```python
from build123d import *

# Parameters (mm, degrees)
SKETCH1_W           = 596.9
SKETCH1_H           = 12.7
BOSS_EXTRUDE1_DEPTH = 6.35
SKETCH3_W           = 37.846
SKETCH3_H           = 6.35
BOSS_EXTRUDE2_DEPTH = 3.175
SKETCH4_R           = 3.429
SKETCH4_R_2         = 4.8895
CUT_EXTRUDE1_DEPTH  = 299.669467179
SKETCH5_R           = 4.9784
CUT_EXTRUDE2_DEPTH  = 299.669467179
CUT_EXTRUDE3_DEPTH  = 299.669467179


with BuildPart() as part:
    # Sketch1 → Boss-Extrude1 (new body)
    with BuildSketch(Plane.XY):
        Rectangle(SKETCH1_W, SKETCH1_H)
    extrude(amount=BOSS_EXTRUDE1_DEPTH)

    # Sketch3 → Boss-Extrude2 (add)
    with BuildSketch(Plane(origin=(0, 6.35, 0), x_dir=(1, 0, 0), z_dir=(0, 1, 0))):
        with Locations((-199.093666667, -3.175)):
            Rectangle(SKETCH3_W, SKETCH3_H)
        with Locations((-99.610333333, -3.175)):
            Rectangle(SKETCH3_W, SKETCH3_H)
        with Locations((-0.127, -3.175)):
            Rectangle(SKETCH3_W, SKETCH3_H)
        with Locations((99.483333333, -3.175)):
            Rectangle(SKETCH3_W, SKETCH3_H)
        with Locations((198.966666751, -3.175)):
            Rectangle(SKETCH3_W, SKETCH3_H)
    boss_extrude2 = extrude(amount=BOSS_EXTRUDE2_DEPTH)

    # Mirror1: Boss-Extrude2 across plane
    add(boss_extrude2.mirror(Plane.ZX))

    # Sketch4 → Cut-Extrude1 (cut, through all)
    with BuildSketch(Plane(origin=(0, 0, 0), x_dir=(-1, 0, 0), z_dir=(0, 0, -1))):
        with Locations((-288.925, 0)):
            Circle(SKETCH4_R)
        with Locations((-244.475, 0)):
            Circle(SKETCH4_R)
        with Locations((-266.7, 0)):
            Circle(SKETCH4_R_2)
    cut_extrude1 = extrude(amount=-CUT_EXTRUDE1_DEPTH, mode=Mode.SUBTRACT)

    # Mirror2: Cut-Extrude1 across plane
    add(cut_extrude1.mirror(Plane(origin=(0, 0, 0), x_dir=(0, 0, 1), z_dir=(1, 0, 0))), mode=Mode.SUBTRACT)

    # Sketch5 → Cut-Extrude2 (cut, through all)
    with BuildSketch(Plane(origin=(0, 0, 0), x_dir=(-1, 0, 0), z_dir=(0, 0, -1))):
        with Locations((-266.7, 0)):
            Circle(SKETCH5_R)
    extrude(amount=-CUT_EXTRUDE2_DEPTH, mode=Mode.SUBTRACT)

    # Sketch6 → Cut-Extrude3 (cut, through all)
    with BuildSketch(Plane.XY.offset(6.35)):
        with BuildLine():
            Line((-208.618666667, 3.81), (-189.568666667, 3.81))
            ThreePointArc((-189.568666667, 3.81), (-185.758666667, 0), (-189.568666667, -3.81))
            Line((-189.568666667, -3.81), (-208.618666667, -3.81))
            ThreePointArc((-208.618666667, -3.81), (-212.428666667, 0), (-208.618666667, 3.81))
        make_face()
        with BuildLine():
            Line((-109.135333333, 3.81), (-90.085333333, 3.81))
            ThreePointArc((-90.085333333, 3.81), (-86.275333333, 0), (-90.085333333, -3.81))
            Line((-90.085333333, -3.81), (-109.135333333, -3.81))
            ThreePointArc((-109.135333333, -3.81), (-112.945333333, 0), (-109.135333333, 3.81))
        make_face()
        with BuildLine():
            Line((-9.652, 3.81), (9.398, 3.81))
            ThreePointArc((9.398, 3.81), (13.208, 0), (9.398, -3.81))
            Line((9.398, -3.81), (-9.652, -3.81))
            ThreePointArc((-9.652, -3.81), (-13.462, 0), (-9.652, 3.81))
        make_face()
        with BuildLine():
            Line((89.831333333, 3.81), (108.881333333, 3.81))
            ThreePointArc((108.881333333, 3.81), (112.691333333, 0), (108.881333333, -3.81))
            Line((108.881333333, -3.81), (89.831333333, -3.81))
            ThreePointArc((89.831333333, -3.81), (86.021333333, 0), (89.831333333, 3.81))
        make_face()
        with BuildLine():
            Line((189.314666667, 3.81), (208.364666667, 3.81))
            ThreePointArc((208.364666667, 3.81), (212.174666667, 0), (208.364666667, -3.81))
            Line((208.364666667, -3.81), (189.314666667, -3.81))
            ThreePointArc((189.314666667, -3.81), (185.504666667, 0), (189.314666667, 3.81))
        make_face()
        with BuildLine():
            Line((-158.877, 3.81), (-139.827, 3.81))
            ThreePointArc((-139.827, 3.81), (-136.017, 0), (-139.827, -3.81))
            Line((-139.827, -3.81), (-158.877, -3.81))
            ThreePointArc((-158.877, -3.81), (-162.687, 0), (-158.877, 3.81))
        make_face()
        with BuildLine():
            Line((-59.319456458, 3.81), (-40.417876875, 3.81))
            ThreePointArc((-40.417876875, 3.81), (-36.607876875, 0), (-40.417876875, -3.81))
            Line((-40.417876875, -3.81), (-59.319456458, -3.81))
            ThreePointArc((-59.319456458, -3.81), (-63.129456458, 0), (-59.319456458, 3.81))
        make_face()
        with BuildLine():
            Line((40.089666667, 3.81), (59.139666667, 3.81))
            ThreePointArc((59.139666667, 3.81), (62.949666667, 0), (59.139666667, -3.81))
            Line((59.139666667, -3.81), (40.089666667, -3.81))
            ThreePointArc((40.089666667, -3.81), (36.279666667, 0), (40.089666667, 3.81))
        make_face()
        with BuildLine():
            Line((139.573, 3.81), (158.623, 3.81))
            ThreePointArc((158.623, 3.81), (162.433, 0), (158.623, -3.81))
            Line((158.623, -3.81), (139.573, -3.81))
            ThreePointArc((139.573, -3.81), (135.763, 0), (139.573, 3.81))
        make_face()
    extrude(amount=-CUT_EXTRUDE3_DEPTH, mode=Mode.SUBTRACT)


solid = part.part
```
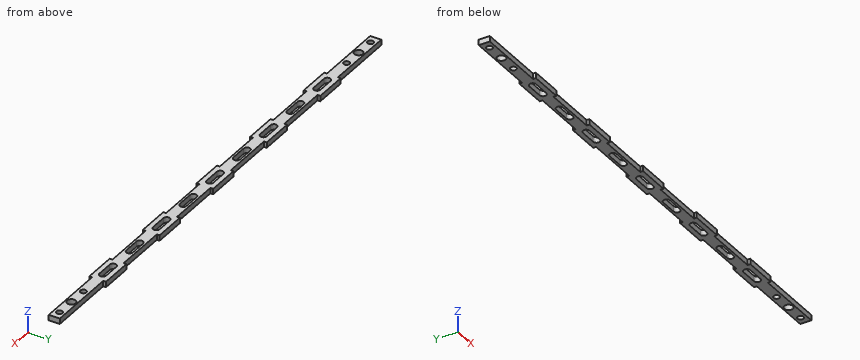
Here's how the part is built. I have some questions about the finished solid (model axes, mm). Coordinates: 2 decimals unless noted, no trailing zeros. Write each loop counter-clockwise with the first axis right and the second up, starting at its lowest first coordinate (ties: lowest second). Pieces come first, ordered by that corner, then holes. Notation, with made-up numbers: (-34.75, 80) -> (-24.75, 80) arc R22 cw to (-24.75, 116) -> close; hole circle Ø5 at (74.25, 8.25). An arc over 180 degrees is marked (long way). Use a Markdown table: item, result. Add a question column.
(1) Please list where these lines run through material, in increasing order: line 1 (Y direction, x = 61, z = 4.5); line 2 (Y direction, x = -244, z = 4); line 3 (Y direction, x = -178, z = 2.25).
(2) If we section it at B-B, the plane x = -266.7: Write out the boundary of the cut face in (y, z), and give its area (3 significant figures).
(3) If we section it at C-C, the plane y = 0: State how many separate pieces and enclosed holes the cut face has, and give its area (3 significant figures).
(4) I'm going to push flat-ended pins straight in: P1, Ø2.5, axis at y = -8.5, z = 4.5, coming from the -X side; P2, Ø6, axis at x = 45, y = -0.5, coming from the -Z side; P3, Ø1.9, axis at x = 51.5, z = 2, coming from the +Y side; P4, Ø2.5, axis at y = -8, z = 3, coming from the +X side. Where does each tip first touch, or does it pass through?
(5) If we section it at A-A, the plane x = 266.7: Write out the boundary of the cut face in (y, z).
Outcome:
| question | item | result |
|---|---|---|
| 1 | line 1 | y = -6.35 to -3.32, 3.32 to 6.35 |
| 1 | line 2 | y = -6.35 to -3.4, 3.4 to 6.35 |
| 1 | line 3 | y = -6.35 to 6.35 |
| 2 | outline | (-6.35, 0) -> (-4.89, 0) -> (-4.89, 6.35) -> (-6.35, 6.35) -> close; (4.89, 0) -> (6.35, 0) -> (6.35, 6.35) -> (4.89, 6.35) -> close |
| 2 | area | 18.5 mm^2 |
| 3 | separate pieces | 16 |
| 3 | enclosed holes | 0 |
| 3 | area | 1,970 mm^2 |
| 4 | P1 | stops at x = -218.02 |
| 4 | P2 | passes through |
| 4 | P3 | stops at y = 6.35 |
| 4 | P4 | stops at x = 217.89 |
| 5 | outline | (-6.35, 0) -> (-4.98, 0) -> (-4.98, 6.35) -> (-6.35, 6.35) -> close; (4.98, 0) -> (6.35, 0) -> (6.35, 6.35) -> (4.98, 6.35) -> close |
